Design review of the part built by this model. Coordinates are the model's own, in mm. Coordinates: 2 decimals unless noted, no trailing zeros. Loops run counter-clockwise (first coordinate to the right, second up) from the corner with the lowest first, then second, coordinate; pieces in that order, holes last. Notation, with made-up numbers: (26, 88) -> (74, 88) arc R21 cw to (74, 119) -> close; hole circle Ø10 at (72.25, 73.25). An arc over 180 degrees is marked (long way). Use a Markdown table: item, result. Add a question column.
Q1. Take a section at D-D on z = 11. Write out the cut boundary in (x, y).
Q2. For probe 1 along X at (y, z) = (3.9, 0); probe 2 along Z at (x, y) = (-3.5, 2.7); probe 3 along X at (y, z) = (3.25, -4.25), list the stretches that pass through material, from the lowest coordinate up.
Q3. Take a section at C-C on y = 2. Count the separate pieces of the cut face and the enclosed holes in it, plus the area to 3 significant figures.
Q4. Draft analysis for pull direction X (two halves, no side actions). For faces 1 (the face through (8.49, 2.56, -3.85)), 2 (the face through (-6, 5.2, 6)), 3 (the face through (4.43, 2.56, 14.07)), state which applies: pulls with the +X half, pulls with the -X half, needs draft (parallel to the pull), parting line crosses it, or undercut.
Q5. Take a section at B-B on z = 0. Write out the cut boundary in (x, y).
Q6. Clearance check with flat-ended pins moving along their axes: pin 1 Ø1 at (y, z) = (2, -4.5) entering from -X; pin 2 Ø1.5 at (x, y) = (-3, 3.5) entering from -Z. State where each tip first meets the part, or that it passes through.
Q7. Take a section at A-A on x = 0. Write out the cut boundary in (y, z), plus the area to 3 significant figures.
from build123d import *

# Parameters (mm, degrees)
SKETCH_1_R               = 14.75
SKETCH_1_R_2             = 7.5
EXTRUDE_1_DEPTH          = 5.2
SKETCH_2_R               = 0.9
CUT_EXTRUDE_1_DEPTH      = 25.266952837
PATTERN_CIRCULAR_1_COUNT = 8


with BuildPart() as part:
    # 草图1 → 凸台-拉伸1 (new body)
    with BuildSketch(Plane(origin=(0, 0, 0), x_dir=(1, 0, 0), z_dir=(0, 1, 0))):
        with Locations(Location((0, 0, 0), (0, 0, 270))):
            Circle(SKETCH_1_R)
        with Locations(Location((0, 0, 0), (0, 0, 270))):
            Circle(SKETCH_1_R_2, mode=Mode.SUBTRACT)
    extrude(amount=EXTRUDE_1_DEPTH)

    # 草图2 → 切除-拉伸1 (cut, through all)
    with BuildSketch(Plane.XZ.offset(7.2)):
        with Locations(Location((9.28608339, -3.430547373, 0), (0, 0, 270))):
            Circle(SKETCH_2_R)
    cut_extrude_1 = extrude(amount=-CUT_EXTRUDE_1_DEPTH, mode=Mode.SUBTRACT)

    # 阵列(圆周)1: 切除-拉伸1 ×8 about axis
    pattern_circular_1_axis = Axis((0, 0, 0), (0, 1, 0))
    for i in range(1, PATTERN_CIRCULAR_1_COUNT):
        add(cut_extrude_1.rotate(pattern_circular_1_axis, i * 360 / PATTERN_CIRCULAR_1_COUNT), mode=Mode.SUBTRACT)


solid = part.part
Answer list:
| question | item | result |
|---|---|---|
| 1 | outline | (-9.83, 0) -> (9.83, 0) -> (9.83, 5.2) -> (-9.83, 5.2) -> close |
| 2 | probe 1 | -14.75 to -7.5, 7.5 to 14.75 |
| 2 | probe 2 | -14.33 to -10.18, -8.39 to -6.63, 6.63 to 8.36, 9.62 to 14.33 |
| 2 | probe 3 | -14.12 to -9.89, -8.1 to -6.18, 6.18 to 8.91, 9.66 to 14.12 |
| 3 | separate pieces | 1 |
| 3 | enclosed holes | 9 |
| 3 | area | 486 mm² |
| 4 | face 1 | undercut |
| 4 | face 2 | needs draft |
| 4 | face 3 | parting line crosses it |
| 5 | outline | (-14.75, 0) -> (-7.5, 0) -> (-7.5, 5.2) -> (-14.75, 5.2) -> close; (7.5, 0) -> (14.75, 0) -> (14.75, 5.2) -> (7.5, 5.2) -> close |
| 6 | pin 1 | x = -14.2 |
| 6 | pin 2 | z = -14.58 |
| 7 | outline | (0, -14.75) -> (5.2, -14.75) -> (5.2, -7.5) -> (0, -7.5) -> close; (0, 7.5) -> (5.2, 7.5) -> (5.2, 14.75) -> (0, 14.75) -> close |
| 7 | area | 75.4 mm² |
